from build123d import *

# Parameters (mm, degrees)
F2_SIZE = 0.5


with BuildPart() as f1:
    # F0 (on Front) → F1 (revolve)
    with BuildSketch(Plane.XZ):
        Polygon((-32.7, 0), (-26.2, 0), (-26.2, 11.4), (-34.7, 11.4), (-34.7, 3.464102), align=None)
    revolve(axis=Axis((0, 0, 86.271172), (0, 0, -1)))

    # F2
    f2_edges = [f1.edges().sort_by_distance(p)[0] for p in [
        (26.2, 0, 11.4),
        (34.7, 0, 11.4),
        (26.2, 0, 0),
    ]]
    chamfer(f2_edges, length=F2_SIZE)


solid = f1.part
CAD build for the part. Positions are in the model's coordinates, mm. Coordinates: 2 decimals unless noted, no trailing zeros. Loops run counter-clockwise (first coordinate to the right, second up) from the corner with the lowest first, then second, coordinate; pieces in that order, holes last. Notation, with made-up numbers: (37.25, 65) - (86.25, 65) arc R20 cw to (86.25, 90) - close; hole circle Ø2 at (87.25, -4). An arc over 180 degrees is marked (long way). Use one line per item in the form item = value. Start each with the question number.
1) Flat gauge pins, fed straight in: pin 1 (3 mm diameter, centred on y = 12, z = 1.5, fed in from -X); pin 2 (2 mm diameter, centred on y = 11, z = 10, fed in from -X); pin 3 (4 mm diameter, centred on y = -4.5, z = 4, fed in from -X). Where does each tip first touch, or does it go through?
2) Drill centre lines: L1, parallel to Y at x = 0, z = 5.5; L2, parallel to Y at x = -20.5, z = 10.25; L3, parallel to X at y = -18, z = 3.25. Where is each one in solid material? Low to high. Write a range as from..to.
3) Band-saw the part on A-A (y = 0). Give the cut face in (x, z).
4) Two-plate mould, pull along X, no slides. Class faces 1 (the face through (20, -18, 11.4)), 2 (the face through (4.517, 34.405, 7.13)), 3 (the face through (3.411, 25.977, 5.773)): +X half, -X half, draft (parallel to the pull), parting line (faces both ways), or undercut.
5) Band-saw the part on C-C (z = 6). Give the cut face in (x, y), and give its area (3 significant figures).
Check values:
q1.pin_1 = -32.42
q1.pin_2 = -33.23
q1.pin_3 = -34.61
q2.L1 = -34.7..-26.2, 26.2..34.7
q2.L2 = -28..-16.32, 16.32..28
q2.L3 = -29.52..-19.04, 19.04..29.52
q3.outline = (-34.7, 3.46) - (-32.7, 0) - (-26.7, 0) - (-26.2, 0.5) - (-26.2, 10.9) - (-26.7, 11.4) - (-34.2, 11.4) - (-34.7, 10.9) - close; (26.2, 0.5) - (26.7, 0) - (32.7, 0) - (34.7, 3.46) - (34.7, 10.9) - (34.2, 11.4) - (26.7, 11.4) - (26.2, 10.9) - close
q4.face_1 = draft
q4.face_2 = parting line
q4.face_3 = undercut
q5.outline = circle Ø69.4 at (0, 0); hole circle Ø52.4 at (0, 0)
q5.area = 1,630 mm2
